For this review, take the finished solid that the model builds, in its own axes (mm). A direction names the side the tool comes from. Coordinates: 2 decimals unless noted, no trailing zeros. Loops run counter-clockwise (first coordinate to the right, second up) from the corner with the lowest first, then second, coordinate; pieces in that order, holes last.
1. Take a section at A-A, the plane y = 43. State the section outline as (x, z) points, then the cut area to 4 significant figures.
2. To check wall thickness, follow probe 1 along Z at (x, y) = (-31.5, 5); probe 2 along Z at (x, y) = (32.5, 16.5). State the ranges of each line that lie inside material, in increasing order.
3. Machinability: for faces 1 (the face through (21, 77, 54)), 2 (the face through (1, 0, -1)), 3 (the face through (-27.6, 31.2, 54.3)), 4 (the face through (-21.06, 25.14, -45.19)), which of the approach directions +Z, -Z, +X, -X, +Y, -Y give a long, thin tool a straight path to every point of the face, cutting with its end or side? Answer none if there is none.
4. Clearance check with flat-ended pins moving along their axes: P1, Ø2, axis at x = -27, y = 78, coming from the -Z side; P2, Ø8, axis at x = 16, y = 16, coming from the +Z side; P3, Ø0.6, axis at y = 23.5, z = 50, coming from the +X side. State where each tip first meets the part, or that it passes through.
5. Mouldability with a two-part tool opening along X and no side actions: class faces 5 (the face through (-50, 49, -1)), 6 (the face through (27.36, 83.94, -45.19)), 7 (the face through (27, 71, 54)) as pulls with the +X half, pulls with the -X half, needs draft (parallel to the pull), parting line crosses it, or undercut.
6. Take a section at B-B, the plane x = -12. State the section outline as (y, z) points, then the cut area to 4 significant figures.
```python
from build123d import *

# Parameters (mm, degrees)
F0_W      = 100
F0_H      = 100
F1_DEPTH  = 100
F2_W      = 20
F2_H      = 20
F3_DEPTH  = 10
F4_SIZE   = 9.5
F5_W      = 20
F5_H      = 20
F6_DEPTH  = 10.25
F7_SIZE   = 9
F8_SIZE   = 0.5
F10_DEPTH = 100


with BuildPart() as f1:
    # F0 (on Front) → F1 (new body, symmetric)
    with BuildSketch(Plane.XZ):
        Rectangle(F0_W, F0_H)
    extrude(amount=F1_DEPTH, both=True)

    # F2 (on face) → F3 (join)
    with BuildSketch(Plane.XY.offset(50)):
        with Locations((-27.5, 77.5)):
            Rectangle(F2_W, F2_H)
        with Locations((27.5, 77.5)):
            Rectangle(F2_W, F2_H)
        with Locations((-27.5, 25)):
            Rectangle(F2_W, F2_H)
        with Locations((-27.5, -25)):
            Rectangle(F2_W, F2_H)
        with Locations((-27.5, -77.5)):
            Rectangle(F2_W, F2_H)
        with Locations((27.5, -77.5)):
            Rectangle(F2_W, F2_H)
        with Locations((27.5, -25)):
            Rectangle(F2_W, F2_H)
        with Locations((27.5, 25)):
            Rectangle(F2_W, F2_H)
    extrude(amount=F3_DEPTH)

    # F4
    f4_edges = [f1.edges().sort_by_distance(p)[0] for p in [
        (27.5, -67.5, 60),
        (17.5, -77.5, 60),
        (27.5, -87.5, 60),
        (37.5, -77.5, 60),
        (27.5, -15, 60),
        (17.5, -25, 60),
        (27.5, -35, 60),
        (37.5, -25, 60),
        (-27.5, -67.5, 60),
        (-37.5, -77.5, 60),
        (-27.5, -87.5, 60),
        (-17.5, -77.5, 60),
        (-27.5, -15, 60),
        (-37.5, -25, 60),
        (-27.5, -35, 60),
        (-17.5, -25, 60),
        (-27.5, 35, 60),
        (-37.5, 25, 60),
        (-27.5, 15, 60),
        (-17.5, 25, 60),
        (-27.5, 87.5, 60),
        (-37.5, 77.5, 60),
        (-27.5, 67.5, 60),
        (-17.5, 77.5, 60),
        (27.5, 87.5, 60),
        (17.5, 77.5, 60),
        (27.5, 67.5, 60),
        (37.5, 77.5, 60),
        (17.5, 25, 60),
        (27.5, 15, 60),
        (37.5, 25, 60),
        (27.5, 35, 60),
    ]]
    chamfer(f4_edges, length=F4_SIZE)

    # F5 (on face) → F6 (cut)
    with BuildSketch(Plane(origin=(0, 0, -50), x_dir=(1, 0, 0), z_dir=(0, 0, -1))):
        with Locations((-27.5, 77.5)):
            Rectangle(F5_W, F5_H)
        with Locations((27.5, 77.5)):
            Rectangle(F5_W, F5_H)
        with Locations((27.5, 25)):
            Rectangle(F5_W, F5_H)
        with Locations((-27.5, 25)):
            Rectangle(F5_W, F5_H)
        with Locations((-27.5, -25)):
            Rectangle(F5_W, F5_H)
        with Locations((27.5, -25)):
            Rectangle(F5_W, F5_H)
        with Locations((27.5, -77.5)):
            Rectangle(F5_W, F5_H)
        with Locations((-27.5, -77.5)):
            Rectangle(F5_W, F5_H)
    extrude(amount=-F6_DEPTH, mode=Mode.SUBTRACT)

    # F7
    f7_edges = [f1.edges().sort_by_distance(p)[0] for p in [
        (27.5, -87.5, -39.75),
        (17.5, -77.5, -39.75),
        (27.5, -67.5, -39.75),
        (37.5, -77.5, -39.75),
        (-27.5, -87.5, -39.75),
        (-37.5, -77.5, -39.75),
        (-27.5, -67.5, -39.75),
        (-17.5, -77.5, -39.75),
        (-27.5, -35, -39.75),
        (-37.5, -25, -39.75),
        (-27.5, -15, -39.75),
        (-17.5, -25, -39.75),
        (17.5, -25, -39.75),
        (27.5, -15, -39.75),
        (37.5, -25, -39.75),
        (27.5, -35, -39.75),
        (27.5, 15, -39.75),
        (17.5, 25, -39.75),
        (27.5, 35, -39.75),
        (37.5, 25, -39.75),
        (-27.5, 15, -39.75),
        (-37.5, 25, -39.75),
        (-27.5, 35, -39.75),
        (-17.5, 25, -39.75),
        (-27.5, 67.5, -39.75),
        (-37.5, 77.5, -39.75),
        (-27.5, 87.5, -39.75),
        (-17.5, 77.5, -39.75),
        (27.5, 67.5, -39.75),
        (17.5, 77.5, -39.75),
        (27.5, 87.5, -39.75),
        (37.5, 77.5, -39.75),
    ]]
    chamfer(f7_edges, length=F7_SIZE)

    # F8
    f8_edges = [f1.edges().sort_by_distance(p)[0] for p in [
        (0, -100, 50),
        (-50, -100, 0),
        (0, -100, -50),
        (50, -100, 0),
        (0, 100, 50),
        (-50, 100, 0),
        (0, 100, -50),
        (50, 100, 0),
        (50, 0, 50),
        (50, 0, -50),
        (-50, 0, 50),
        (-50, 0, -50),
    ]]
    chamfer(f8_edges, length=F8_SIZE)

    # F9 (on face) → F10 (cut)
    with BuildSketch(Plane.YZ.offset(50)):
        Polygon((0, -62.8767311573), (0, 0), (0, 74.2203742266), (-106.3256561756, 74.2203742266), (-106.3256561756, -62.8767311573), align=None)
    extrude(amount=-F10_DEPTH, mode=Mode.SUBTRACT)


solid = f1.part
```
Results list:
1. outline: (-50, -49.5) - (-49.5, -50) - (49.5, -50) - (50, -49.5) - (50, 49.5) - (49.5, 50) - (-49.5, 50) - (-50, 49.5) - close
1. area: 10,000 mm2
2. probe 1: z = -50 to 50
2. probe 2: z = -47.25 to 52
3. face 1: +Z, +Y, -Y
3. face 2: +Z, -Z, +X, -X, -Y
3. face 3: +Z, +X, -X
3. face 4: -Z
4. P1: stops at z = -40.25
4. P2: stops at z = 52.79
4. P3: stops at x = 49.8
5. face 5: pulls with the -X half
5. face 6: undercut
5. face 7: needs draft
6. outline: (0, -50) - (99.5, -50) - (100, -49.5) - (100, 49.5) - (99.5, 50) - (0, 50) - close
6. area: 10,000 mm2
